The model under review builds one solid part; all positions refer to its coordinate system, in mm. A direction names the side the tool comes from. Round coordinates to 2 decimals unless told otherwise and drop trailing zeros. Answer as a JSON object with one key per item and string values. Group by question number.
Item 1: To check wall thickness, follow line 1 (X direction, y = 15, z = -14.5); line 2 (Z direction, x = 15.5, y = 14.5); line 3 (Y direction, x = 7, z = -30). State the ranges of each line that lie inside material, in increasing order.
Item 2: Tool access review of faces 1 (the face through (-3.6, 22.1, -5.8)), 2 (the face through (-17.78, 17, -9)): name each direction out of +Z, -Z, +X, -X, +Y, -Y from which nothing blocks a thin tool from reaching the whole face with its end or side.
Item 3: The part is to be moulded in two halves that separate along Z. For faces 3 (the face through (17.78, 17, -9)), 4 (the face through (-12.7, 33, -27.1)), 5 (the face through (16.794, 10.41, -13.443)), say which applies: +Z half, -Z half, draft (parallel to the pull), parting line (faces both ways), or undercut.
Item 4: Consider section B-B (x = 0). State how many separate pieces and enclosed holes the cut face has, and give its area (3 significant figures).
Item 5: Insertion check: P1, Ø6, axis at x = -9, y = 2, coming from the -Z side; P2, Ø2, axis at x = 12.52, y = -12.52, coming from the +Z side; P3, Ø2, axis at x = 8, y = -14.5, coming from the -Z side; P4, Ø2, axis at x = -10, z = -4, coming from the +Y side. Each pin has a flat end and moves straight along its axis. Give the tip position at first contact, or say it passes through.
```python
from build123d import *

# Parameters (mm, degrees)
SKETCH1_R           = 1.651
SKETCH1_R_2         = 11.07313
BOSS_EXTRUDE1_DEPTH = 2
BOSS_EXTRUDE2_DEPTH = 2
FILLET2_R           = 2
FILLET3_R           = 2


with BuildPart() as part:
    # Sketch1 → Boss-Extrude1 (new body)
    with BuildSketch(Plane.XY):
        with BuildLine():
            Line((-17.78, -10.602028155), (-17.78, 20.701))
            Line((-17.78, 20.701), (17.78, 20.701))
            Line((17.78, 20.701), (17.78, -10.602028155))
            ThreePointArc((17.78, -10.602028155), (0, -20.701), (-17.78, -10.602028155))
        make_face()
        with Locations((-12.515790027, -12.515790027)):
            Circle(SKETCH1_R, mode=Mode.SUBTRACT)
        with Locations((12.515790027, -12.515790027)):
            Circle(SKETCH1_R, mode=Mode.SUBTRACT)
        with Locations((12.515790027, 12.515790027)):
            Circle(SKETCH1_R, mode=Mode.SUBTRACT)
        with Locations((-12.515790027, 12.515790027)):
            Circle(SKETCH1_R, mode=Mode.SUBTRACT)
        Circle(SKETCH1_R_2, mode=Mode.SUBTRACT)
    boss_extrude1 = extrude(amount=BOSS_EXTRUDE1_DEPTH)

    # Mirror1: Boss-Extrude1 across plane
    add(boss_extrude1.mirror(Plane(origin=(0, 13.78083487, -8.816600885), x_dir=(0, 0.5389178124813573, 0.8423583509352233), z_dir=(0, -0.8423583509352232, 0.5389178124813573))))

    # Sketch2 → Boss-Extrude2 (add)
    with BuildSketch(Plane.ZY.offset(17.78)):
        Polygon((0, -10.602028155), (-27.25903588, 32.005352748), (0, 19.421454752), align=None)
    boss_extrude2 = extrude(amount=-BOSS_EXTRUDE2_DEPTH)

    # Mirror2: Boss-Extrude2 across plane
    add(boss_extrude2.mirror(Plane(origin=(0, 0, 0), x_dir=(0, 0, 1), z_dir=(1, 0, 0))))

    # Fillet2
    fillet2_edges = [part.edges().sort_by_distance(p)[0] for p in [
        (-11.07313, 0, 0),
        (-11.07313, 27.561669739, -17.63320177),
    ]]
    fillet(fillet2_edges, radius=FILLET2_R - 0.0001)  # a hair under: the kernel refuses the full size

    # Fillet3
    fillet3_edges = [part.edges().sort_by_distance(p)[0] for p in [
        (-16.78, -10.602028155, 0),
        (-16.78, 32.005352748, -27.25903588),
        (16.78, -10.602028155, 0),
        (16.78, 32.005352748, -27.25903588),
    ]]
    fillet(fillet3_edges, radius=FILLET3_R)


solid = part.part
```
Geometry results:
{
 "1": {"line 1": "x = -17.78 to -15.78, 15.78 to 17.78", "line 2": "z = 0 to 2", "line 3": "y = 33.27 to 35.47"},
 "2": {"face 1": "-Z, -Y", "face 2": "+Z, -Z, -X, +Y, -Y"},
 "3": {"face 3": "draft", "face 4": "undercut", "face 5": "-Z half"},
 "4": {"separate pieces": "3", "enclosed holes": "0", "area": "71.0 mm^2"},
 "5": {"P1": "stops at z = 0.19", "P2": "passes through", "P3": "stops at z = 0", "P4": "stops at y = 23.93"}
}
